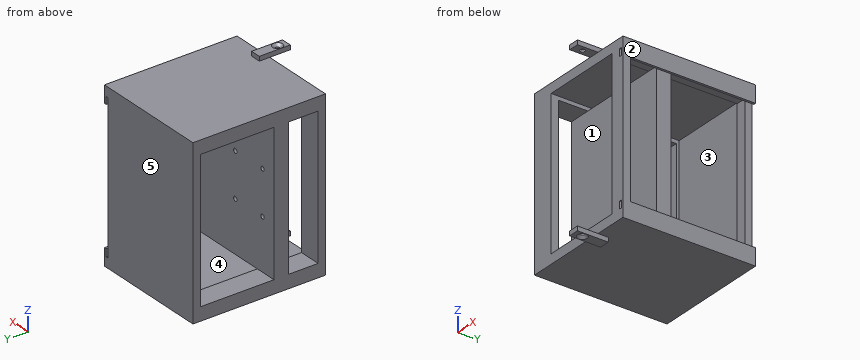
```python
from build123d import *

# Parameters (mm, degrees)
SKETCH1_W                                            = 80
SKETCH1_H                                            = 113
BOSS_EXTRUDE1_DEPTH                                  = 90
SKETCH3_W                                            = 55
SKETCH3_H                                            = 100
CUT_EXTRUDE2_DEPTH                                   = 87
SKETCH4_W                                            = 95
SKETCH4_H                                            = 80
CUT_EXTRUDE3_DEPTH                                   = 77
SKETCH6_W                                            = 95
SKETCH6_H                                            = 10
BOSS_EXTRUDE4_DEPTH                                  = 77
CUT_EXTRUDE4_DEPTH                                   = 91
F_3_0_3_DIAMETER_HOLE1_D                             = 3
F_3_0_3_DIAMETER_HOLE1_DEPTH                         = 5.098709071
F_3_0_3_DIAMETER_HOLE1_CSINK_D                       = 3.05
F_3_0_3_DIAMETER_HOLE1_CSINK_ANGLE                   = 90
F_3_0_3_DIAMETER_HOLE1_TIP                           = 0.901290929
SKETCH11_W                                           = 90
SKETCH11_H                                           = 5
BOSS_EXTRUDE5_DEPTH                                  = 3
SKETCH12_W                                           = 7
SKETCH12_H                                           = 21
BOSS_EXTRUDE6_DEPTH                                  = 3
SKETCH13_W                                           = 7
SKETCH13_H                                           = 21
BOSS_EXTRUDE7_DEPTH                                  = 3
CSK_FOR_M3_HEX_SOCKET_COUNTERSUNK_CAP_SC_D           = 3.2
CSK_FOR_M3_HEX_SOCKET_COUNTERSUNK_CAP_SC_DEPTH       = 7.23862301
CSK_FOR_M3_HEX_SOCKET_COUNTERSUNK_CAP_SC_CSINK_D     = 6.72
CSK_FOR_M3_HEX_SOCKET_COUNTERSUNK_CAP_SC_CSINK_ANGLE = 90
CSK_FOR_M3_HEX_SOCKET_COUNTERSUNK_CAP_SC_TIP         = 0.96137699
CSK_FOR_M3_HEX_SOCKET_COUNTERSUNK_CA_2_D             = 3.2
CSK_FOR_M3_HEX_SOCKET_COUNTERSUNK_CA_2_DEPTH         = 7.23862301
CSK_FOR_M3_HEX_SOCKET_COUNTERSUNK_CA_2_CSINK_D       = 6.72
CSK_FOR_M3_HEX_SOCKET_COUNTERSUNK_CA_2_CSINK_ANGLE   = 90
CSK_FOR_M3_HEX_SOCKET_COUNTERSUNK_CA_2_TIP           = 0.96137699


with BuildPart() as part:
    # Sketch1 → Boss-Extrude1 (new body)
    with BuildSketch(Plane(origin=(0, 0, 0), x_dir=(1, 0, 0), z_dir=(0, 1, 0))):
        Rectangle(SKETCH1_W, SKETCH1_H)
    extrude(amount=BOSS_EXTRUDE1_DEPTH)

    # Sketch3 → Cut-Extrude2 (cut)
    with BuildSketch(Plane.XZ):
        with Locations((2.5, 0)):
            Rectangle(SKETCH3_W, SKETCH3_H)
    extrude(amount=-CUT_EXTRUDE2_DEPTH, mode=Mode.SUBTRACT)

    # Sketch4 → Cut-Extrude3 (cut)
    with BuildSketch(Plane.ZY.offset(40)):
        with Locations((0, 45)):
            Rectangle(SKETCH4_W, SKETCH4_H)
    extrude(amount=-CUT_EXTRUDE3_DEPTH, mode=Mode.SUBTRACT)

    # Sketch6 → Boss-Extrude4 (add)
    with BuildSketch(Plane.ZY.offset(-37)):
        with Locations((0, 30)):
            Rectangle(SKETCH6_W, SKETCH6_H)
    extrude(amount=BOSS_EXTRUDE4_DEPTH)

    # Sketch7 → Cut-Extrude4 (cut, through all)
    with BuildSketch(Plane(origin=(0, 0, 0), x_dir=(1, 0, 0), z_dir=(0, 1, 0))):
        Polygon((40, 45), (38.5, 45), (38.5, 50), (37, 50), (37, -50), (38.5, -50), (38.5, -45), (40, -45), align=None)
    extrude(amount=CUT_EXTRUDE4_DEPTH, mode=Mode.SUBTRACT)

    # Ø3.0 (3) Diameter Hole1
    with Locations(Plane(origin=(0, 35, 0), x_dir=(1, 0, 0), z_dir=(0, 1, 0))):
        with Locations((-5.02, -17.05), (-5.02, 12.84), (-29.68, 12.84), (-29.68, -17.05)):
            CounterSinkHole(F_3_0_3_DIAMETER_HOLE1_D / 2, F_3_0_3_DIAMETER_HOLE1_CSINK_D / 2, depth=F_3_0_3_DIAMETER_HOLE1_DEPTH, counter_sink_angle=F_3_0_3_DIAMETER_HOLE1_CSINK_ANGLE)
            with Locations((0, 0, -(F_3_0_3_DIAMETER_HOLE1_DEPTH + F_3_0_3_DIAMETER_HOLE1_TIP / 2))):  # 118° drill point
                Cone(0, F_3_0_3_DIAMETER_HOLE1_D / 2, F_3_0_3_DIAMETER_HOLE1_TIP, mode=Mode.SUBTRACT)

    # Sketch11 → Boss-Extrude5 (add, through all)
    with BuildSketch(Plane(origin=(37, 0, 0), x_dir=(0, 0, -1), z_dir=(1, 0, 0))):
        with Locations((0, 2.5)):
            Rectangle(SKETCH11_W, SKETCH11_H)
    extrude(amount=BOSS_EXTRUDE5_DEPTH)

    # Sketch12 → Boss-Extrude6 (add)
    with BuildSketch(Plane.XY.offset(56.5)):
        with Locations((14, -3.5)):
            Rectangle(SKETCH12_W, SKETCH12_H)
    extrude(amount=BOSS_EXTRUDE6_DEPTH)

    # Sketch13 → Boss-Extrude7 (add)
    with BuildSketch(Plane(origin=(0, 0, -56.5), x_dir=(-1, 0, 0), z_dir=(0, 0, -1))):
        with Locations((-14, -3.5)):
            Rectangle(SKETCH13_W, SKETCH13_H)
    extrude(amount=BOSS_EXTRUDE7_DEPTH)

    # CSK for M3 Hex Socket Countersunk Cap Sc
    with Locations(Plane(origin=(0, 0, -59.5), x_dir=(-1, 0, 0), z_dir=(0, 0, -1))):
        with Locations((-14, -8)):
            CounterSinkHole(CSK_FOR_M3_HEX_SOCKET_COUNTERSUNK_CAP_SC_D / 2, CSK_FOR_M3_HEX_SOCKET_COUNTERSUNK_CAP_SC_CSINK_D / 2, depth=CSK_FOR_M3_HEX_SOCKET_COUNTERSUNK_CAP_SC_DEPTH, counter_sink_angle=CSK_FOR_M3_HEX_SOCKET_COUNTERSUNK_CAP_SC_CSINK_ANGLE)
            with Locations((0, 0, -(CSK_FOR_M3_HEX_SOCKET_COUNTERSUNK_CAP_SC_DEPTH + CSK_FOR_M3_HEX_SOCKET_COUNTERSUNK_CAP_SC_TIP / 2))):  # 118° drill point
                Cone(0, CSK_FOR_M3_HEX_SOCKET_COUNTERSUNK_CAP_SC_D / 2, CSK_FOR_M3_HEX_SOCKET_COUNTERSUNK_CAP_SC_TIP, mode=Mode.SUBTRACT)

    # CSK for M3 Hex Socket Countersunk Ca 2
    with Locations(Plane.XY.offset(59.5)):
        with Locations((14, -8)):
            CounterSinkHole(CSK_FOR_M3_HEX_SOCKET_COUNTERSUNK_CA_2_D / 2, CSK_FOR_M3_HEX_SOCKET_COUNTERSUNK_CA_2_CSINK_D / 2, depth=CSK_FOR_M3_HEX_SOCKET_COUNTERSUNK_CA_2_DEPTH, counter_sink_angle=CSK_FOR_M3_HEX_SOCKET_COUNTERSUNK_CA_2_CSINK_ANGLE)
            with Locations((0, 0, -(CSK_FOR_M3_HEX_SOCKET_COUNTERSUNK_CA_2_DEPTH + CSK_FOR_M3_HEX_SOCKET_COUNTERSUNK_CA_2_TIP / 2))):  # 118° drill point
                Cone(0, CSK_FOR_M3_HEX_SOCKET_COUNTERSUNK_CA_2_D / 2, CSK_FOR_M3_HEX_SOCKET_COUNTERSUNK_CA_2_TIP, mode=Mode.SUBTRACT)


solid = part.part
```
Can you work these out from the model? Positions are in its coordinate system, mm. Face numbers are marked on the shaded views. A direction names the side the tool comes from. Round coordinates to 2 decimals unless told otherwise and drop trailing zeros. Order: outer loops, then holes, each group sorted by start corner. A loop starts at its lowest first (then second) coordinate and runs counter-clockwise, first axis right, second up. Notation, with made-up numbers: (-36.5, 58.5) -> (18.5, 58.5) arc R25 cw to (18.5, 85.5) -> close; hole circle Ø2 at (73.5, 75). An arc over 180 degrees is marked (long way). Return JSON: item names as keys, results as strings. Group by question number.
1. We'd pull the mould along Z, two halves only. Please class the marked faces 1 and 2: released by +Z, released by -Z, zero draft, split by the parting line, or undercut.
2. Which directions (+Z, -Z, +X, -X, +Y, -Y) give clear straight access to the entire face, cutting with the end or side of a thin tool? Please do the marked faces 3, 4 and 5.
3. If we section it at C-C, the plane z = 25: Write out the boundary of the cut face in (x, y), then the cut area to 3 significant figures.
4. If we section it at D-D, the plane y = -8: Write out the boundary of the cut face in (x, z), then the cut area to 3 significant figures.
5. If we section it at B-B, the plane y = 46.5: Write out the boundary of the cut face in (x, z).
6. Will these pins go through, and if not, where does the flat tip stop? pin 1 (2.5 mm diameter, centred on x = -29.68, z = -12.84, fed in from -Y); pin 2 (1.6 mm diameter, centred on x = 39, y = 28.5, fed in from +Z); pin 3 (23 mm diameter, centred on x = -12, z = -18, fed in from -Y).
7. I need wall thicknesses on line 1 (Z direction, x = -29.68, y = 31.3); line 2 (X direction, y = 32.7, z = -12.84); line 3 (Y direction, x = 30.5, z = -41.5). Which ranges of each line are inside material? Lowest first, please. Write a range as [from, to].
8. If we section it at A-A, the plane x = 14: Count the separate pieces of the cut face and the enclosed holes in it, then the cut area to 3 significant figures.
Output values:
{
 "1": {"face 1": "undercut", "face 2": "zero draft"},
 "2": {"face 3": "none", "face 4": "-Y", "face 5": "+Z, -Z, +X, -X, +Y"},
 "3": {"outline": "(-40, 0) -> (-25, 0) -> (-25, 5) -> (-40, 5) -> close; (-40, 25) -> (37, 25) -> (37, 35) -> (-40, 35) -> close; (-40, 85) -> (-25, 85) -> (-25, 87) -> (30, 87) -> (30, 85) -> (37, 85) -> (37, 90) -> (-40, 90) -> close; (30, 0) -> (40, 0) -> (40, 5) -> (30, 5) -> close", "area": "1,170 mm²"},
 "4": {"outline": "(10.5, -59.5) -> (10.64, -59.5) -> (12.4, -57.74) -> (12.4, -56.5) -> (10.5, -56.5) -> close; (10.5, 56.5) -> (12.4, 56.5) -> (12.4, 57.74) -> (10.64, 59.5) -> (10.5, 59.5) -> close; (15.6, -57.74) -> (17.36, -59.5) -> (17.5, -59.5) -> (17.5, -56.5) -> (15.6, -56.5) -> close; (15.6, 56.5) -> (17.5, 56.5) -> (17.5, 59.5) -> (17.36, 59.5) -> (15.6, 57.74) -> close", "area": "16.6 mm²"},
 "5": {"outline": "(-40, -56.5) -> (40, -56.5) -> (40, -45) -> (38.5, -45) -> (38.5, -50) -> (37, -50) -> (37, -47.5) -> (30, -47.5) -> (30, -50) -> (-25, -50) -> (-25, -47.5) -> (-40, -47.5) -> close; (-40, 47.5) -> (-25, 47.5) -> (-25, 50) -> (30, 50) -> (30, 47.5) -> (37, 47.5) -> (37, 50) -> (38.5, 50) -> (38.5, 45) -> (40, 45) -> (40, 56.5) -> (-40, 56.5) -> close"},
 "6": {"pin 1": "y = 0", "pin 2": "z = 56.5", "pin 3": "y = 25"},
 "7": {"line 1": "[-56.5, -14.34], [-11.34, 15.55], [18.55, 56.5]", "line 2": "[-40, -31.18], [-28.18, -6.52], [-3.52, 37]", "line 3": "[0, 5], [25, 35], [85, 90]"},
 "8": {"separate pieces": "4", "enclosed holes": "0", "area": "2,520 mm²"}
}
